Input: part model. Units: mm. Frame: model coordinates. Face numbers are marked on the shaded views. Coordinates: 2 decimals unless noted, no trailing zeros. Write each loop counter-clockwise with the first axis right and the second up, starting at its lowest first coordinate (ties: lowest second). Pieces come first, ordered by that corner, then holes. Notation, with made-up numbers: (37.5, 43) - (49.5, 43) arc R4 cw to (49.5, 48) - close; hole circle Ø7 at (-28.5, 48). An arc over 180 degrees is marked (long way). Put each result on its own line as item: value. Start each with the question number.
1. Pull-direction query (X, two-part tool) for the marked faces 1, 2 and 3; classes: released by +X, released by -X, zero draft, split by the parting line, or undercut.
2. Cut plane D-D, the plane z = 1.1. Return loops of the section in (x, y).
3. Cut plane A-A, the plane z = 0. Return loops of the section in (x, y), and give its area (3 significant figures).
4. Cut plane C-C, the plane y = 2.9. Return loops of the section in (x, z), and give its area (3 significant figures).
5. Cut plane B-B, the plane x = -10. Return loops of the section in (y, z), and give its area (3 significant figures).
6. Line query: line 1 (X direction, y = 1.65, z = 0); line 2 (X direction, y = 3.9, z = 1.55); line 3 (Z direction, x = 10, y = 2.25). Output: solid intervals per line, ascending.
from build123d import *

# Parameters (mm, degrees)
ESQUISSE1_W          = 30
ESQUISSE1_H          = 6
BOSS_EXTRU_1_DEPTH   = 5
D_GAGEMENT_M31_D     = 3.4
D_GAGEMENT_M31_DEPTH = 5
D_GAGEMENT_M31_TIP   = 1.021463052


with BuildPart() as part:
    # Esquisse1 → Boss.-Extru.1 (new body)
    with BuildSketch(Plane(origin=(0, 0, 0), x_dir=(1, 0, 0), z_dir=(0, 1, 0))):
        Rectangle(ESQUISSE1_W, ESQUISSE1_H)
    extrude(amount=BOSS_EXTRU_1_DEPTH)

    # Dégagement M31
    with Locations(Plane.XZ):
        with Locations((10, 0), (-10, 0)):
            Hole(D_GAGEMENT_M31_D / 2, depth=D_GAGEMENT_M31_DEPTH)
            with Locations((0, 0, -(D_GAGEMENT_M31_DEPTH + D_GAGEMENT_M31_TIP / 2))):  # 118° drill point
                Cone(0, D_GAGEMENT_M31_D / 2, D_GAGEMENT_M31_TIP, mode=Mode.SUBTRACT)


solid = part.part
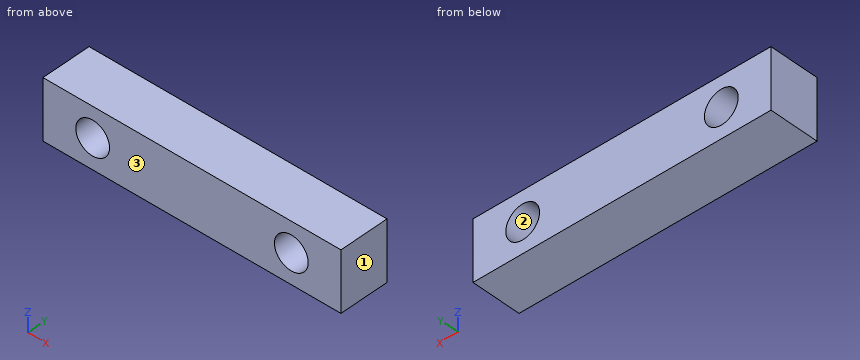
Report:
1. face 1: released by +X
1. face 2: undercut
1. face 3: zero draft
2. outline: (-15, 0) - (-11.3, 0) - (-11.3, 5) - (-15, 5) - close; (-8.7, 0) - (8.7, 0) - (8.7, 5) - (-8.7, 5) - close; (11.3, 0) - (15, 0) - (15, 5) - (11.3, 5) - close
3. outline: (-15, 0) - (-11.7, 0) - (-11.7, 5) - (-15, 5) - close; (-8.3, 0) - (8.3, 0) - (8.3, 5) - (-8.3, 5) - close; (11.7, 0) - (15, 0) - (15, 5) - (11.7, 5) - close
3. area: 116 mm^2
4. outline: (-15, -3) - (15, -3) - (15, 3) - (-15, 3) - close; hole circle Ø3.4 at (-10, 0); hole circle Ø3.4 at (10, 0)
4. area: 162 mm^2
5. outline: (0, -3) - (5, -3) - (5, -1.7) - (0, -1.7) - close; (0, 1.7) - (5, 1.7) - (5, 3) - (0, 3) - close
5. area: 13.0 mm^2
6. line 1: x = -15 to -11.7, -8.3 to 8.3, 11.7 to 15
6. line 2: x = -15 to -10.7, -9.3 to 9.3, 10.7 to 15
6. line 3: z = -3 to -1.7, 1.7 to 3
